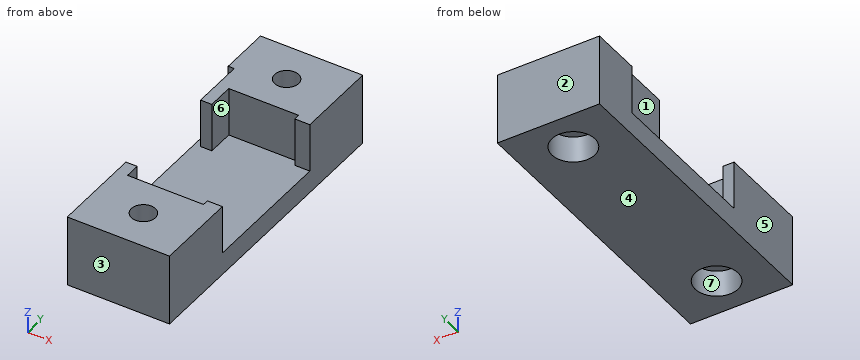
from build123d import *

# Parameters (mm, degrees)
SKETCH1_R               = 2.85
SKETCH1_R_2             = 1.6
BOSS_EXTRUDE1_DEPTH     = 6.5
SKETCH1_3_R             = 2.85
SKETCH1_3_R_2           = 1.6
BOSS_EXTRUDE2_DEPTH     = 3
CUT_EXTRUDE1_START      = -3
SKETCH1_4_R             = 2.85
CUT_EXTRUDE1_DEPTH      = 3.5
CUT_EXTRUDE1_DEPTH_BACK = 4


with BuildPart() as part:
    # Sketch1 → Boss-Extrude1 (new body)
    with BuildSketch(Plane(origin=(0, 0, 0), x_dir=(0, 1, 0), z_dir=(0, 0, 1))):
        Polygon((-7.9, 10.1), (-9.9, 10.1), (-9.9, 0), (-9.1, 0), (-9.1, -2), (-20.1, -2), (-20.1, 11.6), (-7.9, 11.6), align=None)
        with Locations((-14.9, 4.8)):
            Circle(SKETCH1_R, mode=Mode.SUBTRACT)
        Polygon((13.378898747, 11.6), (20.1, 11.6), (20.1, -2), (9.1, -2), (9.1, 0), (9.9, 0), (9.9, 9.3), (6.378898747, 9.3), (6.378898747, 10.8), (13.378898747, 10.8), align=None)
        with Locations((14.9, 4.8)):
            Circle(SKETCH1_R, mode=Mode.SUBTRACT)
        with Locations((-14.9, 4.8)):
            Circle(SKETCH1_R)
        with Locations((-14.9, 4.8)):
            Circle(SKETCH1_R_2, mode=Mode.SUBTRACT)
        with Locations((14.9, 4.8)):
            Circle(SKETCH1_R)
        with Locations((14.9, 4.8)):
            Circle(SKETCH1_R_2, mode=Mode.SUBTRACT)
    extrude(amount=BOSS_EXTRUDE1_DEPTH)

    # Sketch1<3> → Boss-Extrude2 (add)
    with BuildSketch(Plane(origin=(0, 0, 0), x_dir=(0, 1, 0), z_dir=(0, 0, 1))):
        with Locations((14.9, 4.8)):
            Circle(SKETCH1_3_R)
        with Locations((14.9, 4.8)):
            Circle(SKETCH1_3_R_2, mode=Mode.SUBTRACT)
        Polygon((13.378898747, 11.6), (20.1, 11.6), (20.1, -2), (9.1, -2), (9.1, 0), (9.9, 0), (9.9, 9.3), (6.378898747, 9.3), (6.378898747, 10.8), (13.378898747, 10.8), align=None)
        with Locations((14.9, 4.8)):
            Circle(SKETCH1_3_R, mode=Mode.SUBTRACT)
        Polygon((-7.9, 11.6), (13.378898747, 11.6), (13.378898747, 10.8), (6.378898747, 10.8), (6.378898747, 9.3), (9.9, 9.3), (9.9, 0), (9.1, 0), (9.1, -2), (-9.1, -2), (-9.1, 0), (-9.9, 0), (-9.9, 10.1), (-7.9, 10.1), align=None)
        with Locations((-14.9, 4.8)):
            Circle(SKETCH1_3_R)
        with Locations((-14.9, 4.8)):
            Circle(SKETCH1_3_R_2, mode=Mode.SUBTRACT)
        Polygon((-7.9, 10.1), (-9.9, 10.1), (-9.9, 0), (-9.1, 0), (-9.1, -2), (-20.1, -2), (-20.1, 11.6), (-7.9, 11.6), align=None)
        with Locations((-14.9, 4.8)):
            Circle(SKETCH1_3_R, mode=Mode.SUBTRACT)
    extrude(amount=-BOSS_EXTRUDE2_DEPTH)

    # Sketch1<4> → Cut-Extrude1 (cut, two sides)
    with BuildSketch(Plane(origin=(0, 0, 0), x_dir=(0, 1, 0), z_dir=(0, 0, 1)).offset(CUT_EXTRUDE1_START)) as cut_extrude1_sk:
        with Locations((14.9, 4.8)):
            Circle(SKETCH1_4_R)
        with Locations((-14.9, 4.8)):
            Circle(SKETCH1_4_R)
    extrude(amount=CUT_EXTRUDE1_DEPTH, mode=Mode.SUBTRACT)
    extrude(cut_extrude1_sk.sketch, amount=-CUT_EXTRUDE1_DEPTH_BACK, mode=Mode.SUBTRACT)


solid = part.part
Can you work these out from the model? Positions are in its coordinate system, mm. Face numbers are marked on the shaded views. A direction names the side the tool comes from. Round coordinates to 2 decimals unless told otherwise and drop trailing zeros. Write each loop counter-clockwise with the first axis right and the second up, starting at its lowest first coordinate (ties: lowest second). Pieces come first, ordered by that corner, then holes. Notation, with made-up numbers: M 69,86.25 L 115,86.25 A12 cw 115,97.25 Z; hole C -23,35.25 d1. An arc over 180 degrees is marked long. Use a Markdown table: item, result.
Item 1: I want a section at B-B (y = 14.9). List the corners of the cut face in (x, z) for me, and give its area (4 significant figures).
Found:
| item | result |
|---|---|
| outline | M -11.6,-3 L -7.65,-3 L -7.65,0.5 L -6.4,0.5 L -6.4,6.5 L -11.6,6.5 Z; M -3.2,0.5 L -1.95,0.5 L -1.95,-3 L 2,-3 L 2,6.5 L -3.2,6.5 Z |
| area | 90.05 mm2 |
Item 2: I want a section at A-A (z = 1.75). List the corners of the cut face in (x, y) for me.
Found:
| item | result |
|---|---|
| outline | M -11.6,-20.1 L 2,-20.1 L 2,-9.1 L 0,-9.1 L 0,-9.9 L -10.1,-9.9 L -10.1,-7.9 L -11.6,-7.9 Z; M -11.6,13.38 L -10.8,13.38 L -10.8,6.38 L -9.3,6.38 L -9.3,9.9 L 0,9.9 L 0,9.1 L 2,9.1 L 2,20.1 L -11.6,20.1 Z; hole C -4.8,-14.9 d3.2; hole C -4.8,14.9 d3.2 |
Item 3: We'd pull the mould along Y, two halves only. Please class the marked faces 1, 2, 3 and 4: released by +Y, released by -Y, zero draft, split by the parting line, or undercut.
Found:
| item | result |
|---|---|
| face 1 | undercut |
| face 2 | released by +Y |
| face 3 | released by -Y |
| face 4 | zero draft |
Item 4: I want a section at C-C (x = -4.8). List the corners of the cut face in (y, z) for me.
Found:
| item | result |
|---|---|
| outline | M -20.1,-3 L -17.75,-3 L -17.75,0.5 L -16.5,0.5 L -16.5,6.5 L -20.1,6.5 Z; M -13.3,0.5 L -12.05,0.5 L -12.05,-3 L 12.05,-3 L 12.05,0.5 L 13.3,0.5 L 13.3,6.5 L 9.9,6.5 L 9.9,0 L -9.9,0 L -9.9,6.5 L -13.3,6.5 Z; M 16.5,0.5 L 17.75,0.5 L 17.75,-3 L 20.1,-3 L 20.1,6.5 L 16.5,6.5 Z |
Item 5: I want a section at D-D (y = 7.5). List the corners of the cut face in (x, z) for me.
Found:
| item | result |
|---|---|
| outline | M -11.6,-3 L 2,-3 L 2,0 L -9.3,0 L -9.3,6.5 L -10.8,6.5 L -10.8,0 L -11.6,0 Z |
Item 6: Which directions (+Z, -Z, +X, -X, +Y, -Y) give clear straight access to the entire face, cutting with the end or side of a thin tool? Please do the marked faces 5, 6 and 7.
Found:
| item | result |
|---|---|
| face 5 | +Z, -Z, -X, +Y, -Y |
| face 6 | +Z |
| face 7 | -Z |
Item 7: For pin 1 Ø3.5 at (x, y) = (-4.8, -14.9) entering from -Z; pin 2 Ø6 at (x, y) = (-5, 3) entering from +Z, each with a flat end and sliding along its axis, tell me the tip position at first contact or that it passes through.
Found:
| item | result |
|---|---|
| pin 1 | stops at z = 0.5 |
| pin 2 | stops at z = 0 |
Item 8: If I drill on line 1 along Y through (x, z) = (-4.8, -1.05); line 2 along Y through (x, z) = (-4.8, 3.6); line 3 along Y through (x, z) = (-3.5, 4.25), over which ranges is the centre line in solid material (lowest first)? Write a range as [from, to].
Found:
| item | result |
|---|---|
| line 1 | y = [-20.1, -17.75], [-12.05, 12.05], [17.75, 20.1] |
| line 2 | y = [-20.1, -16.5], [-13.3, -9.9], [9.9, 13.3], [16.5, 20.1] |
| line 3 | y = [-20.1, -15.83], [-13.97, -9.9], [9.9, 13.97], [15.83, 20.1] |
